Here's how the part is built. I have some questions about the finished solid (model axes, mm). A direction names the side the tool comes from. Round coordinates to 2 decimals unless told otherwise and drop trailing zeros. Write each loop counter-clockwise with the first axis right and the second up, starting at its lowest first coordinate (ties: lowest second). Pieces come first, ordered by that corner, then holes. Notation, with made-up numbers: (4, -22.75) - (9, -22.75) arc R22 cw to (9, -4.75) - close; hole circle Ø11 at (81, -21). An arc over 180 degrees is marked (long way). One line per question, with ' | ' between items. Start each with the question number.
(1) Will these pins go through, and if not, where does the flat tip stop? pin 1 (1.7 mm diameter, centred on x = -20.5, y = 5, fed in from +Z); pin 2 (3.5 mm diameter, centred on y = 4, z = -21.5, fed in from -X); pin 3 (4 mm diameter, centred on x = -10, y = 2, fed in from -Z); pin 4 (1 mm diameter, centred on y = 2, z = -21.5, fed in from +X).
(2) Imagine slicing it at B-B (y = 3.5). Write out the boundary of the cut face in (x, z).
(3) For faces 1 (the flat face through (-6, 0, -14)), 2 (the flat face through (0, 4, 19)), 3 (the flat face through (-20, 4, 2.5)), 4 (the flat face through (0, 4, -19)), 5 (the flat face through (19, 4, 0)), which set-ups out of +Z, -Z, +X, -X, +Y, -Y let a thin tool reach every point of the face, with its end or its side?
(4) If I drill on L1, parallel to X at y = 3.75, z = 0; L2, parallel to X at y = 5, z = 11; L3, parallel to Z at x = -6.5, y = 5.25, over which ranges is the centre line in solid material (lowest first)?
(5) Thinking about a two-plate mould opening in Z: for faces 6 (the flat face through (-20, 4, -2.5)), 7 (the flat face through (2.5, 4, 20)), 8 (the cylindrical face through (16.06, 5.61, 15.76)), which applies, pulls with the +Z half, pulls with the -Z half, needs draft (parallel to the pull), parting line crosses it, or undercut?
(6) Imagine slicing it at A-A (y = 6.25). Write out the boundary of the cut face in (x, z).
from build123d import *

# Parameters (mm, degrees)
NOTCH_DEPTH       = 33.580669115
CIRPATTERN1_COUNT = 4


with BuildPart() as part:
    # Profile → Nut (revolve)
    with BuildSketch(Plane.XY, mode=Mode.PRIVATE) as nut_sk:
        Polygon((15, 7), (15, 0), (19, 0), (22.5, 4.171137574), (22.5, 7), align=None)
    revolve(nut_sk.sketch.rotate(Axis((0, 25.4, 0), (0, -1, 0)), 90), axis=Axis((0, 25.4, 0), (0, -1, 0)))

    # Cut → Notch (cut, through all)
    with BuildSketch(Plane(origin=(0, 7, 0), x_dir=(-1, 0, 0), z_dir=(0, 1, 0))):
        with BuildLine():
            Line((2.5, -19), (-2.5, -19))
            Line((-2.5, -19), (-2.5, -22.360679775))
            ThreePointArc((-2.5, -22.360679775), (0, -22.5), (2.5, -22.360679775))
            Line((2.5, -22.360679775), (2.5, -19))
        make_face()
    notch = extrude(amount=-NOTCH_DEPTH, mode=Mode.SUBTRACT)

    # CirPattern1: Notch ×4 about axis
    cirpattern1_axis = Axis((0, 0, 0), (0, 1, 0))
    for i in range(1, CIRPATTERN1_COUNT):
        add(notch.rotate(cirpattern1_axis, i * 360 / CIRPATTERN1_COUNT), mode=Mode.SUBTRACT)


solid = part.part
Check sheet entries:
1) pin 1: z = 10.96 | pin 2: x = -10.76 | pin 3: z = -20.22 | pin 4: through
2) outline: (-21.79, -2.5) arc R21.94 ccw to (-2.5, -21.79) - (-2.5, -19) - (2.5, -19) - (2.5, -21.79) arc R21.94 ccw to (21.79, -2.5) - (19, -2.5) - (19, 2.5) - (21.79, 2.5) arc R21.94 ccw to (2.5, 21.79) - (2.5, 19) - (-2.5, 19) - (-2.5, 21.79) arc R21.94 ccw to (-21.79, 2.5) - (-19, 2.5) - (-19, -2.5) - close; hole circle Ø30 at (0, 0)
3) face 1: +Z, -Z, +X, -X, -Y | face 2: +Z, +Y, -Y | face 3: -X, +Y, -Y | face 4: -Z, +Y, -Y | face 5: +X, +Y, -Y
4) L1: -19 to -15, 15 to 19 | L2: -19.63 to -10.2, 10.2 to 19.63 | L3: -21.54 to -13.52, 13.52 to 21.54
5) face 6: undercut | face 7: needs draft | face 8: pulls with the +Z half
6) outline: (-22.36, -2.5) arc R22.5 ccw to (-2.5, -22.36) - (-2.5, -19) - (2.5, -19) - (2.5, -22.36) arc R22.5 ccw to (22.36, -2.5) - (19, -2.5) - (19, 2.5) - (22.36, 2.5) arc R22.5 ccw to (2.5, 22.36) - (2.5, 19) - (-2.5, 19) - (-2.5, 22.36) arc R22.5 ccw to (-22.36, 2.5) - (-19, 2.5) - (-19, -2.5) - close; hole circle Ø30 at (0, 0)
